Verification items for this drawing (mm, ordinates from the low corner). Coordinates: 2 decimals unless noted, no trailing zeros. Write each loop counter-clockwise with the first axis right and the second up, starting at its lowest first coordinate (ties: lowest second). Pieces come first, ordered by that corner, then holes.
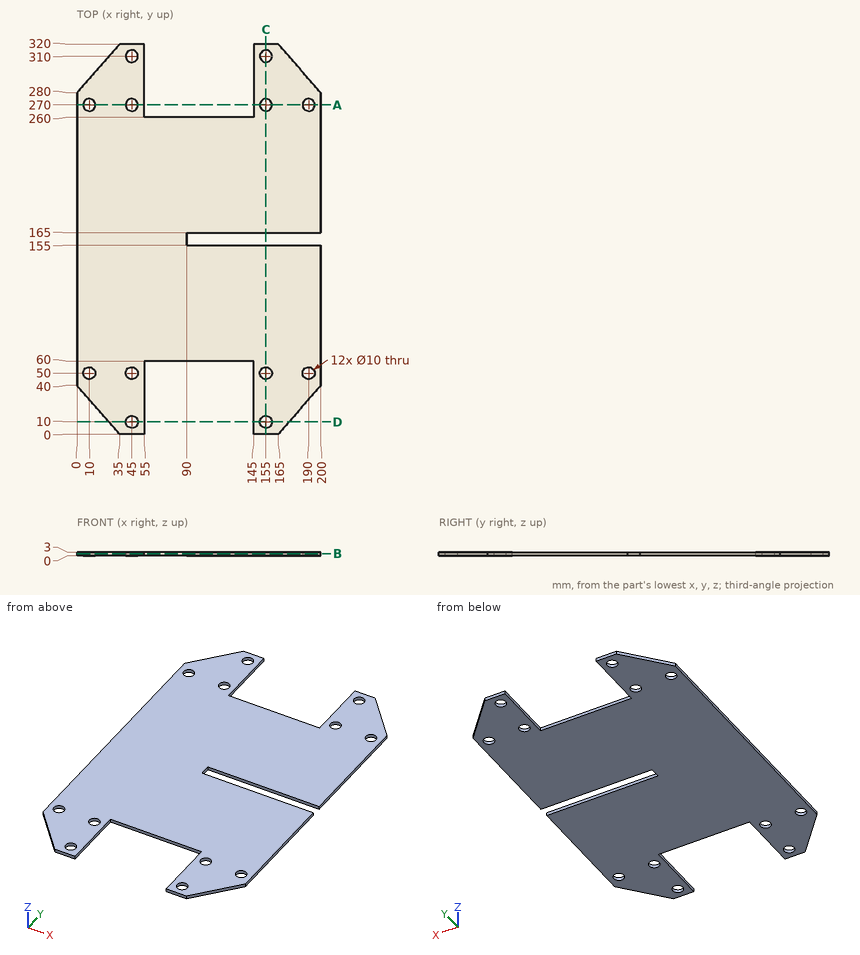
1. Sectioned sample at D-D, the plane y = 10. Record the boundary of the cut face in (x, z).
Computed values:
outline: (26.25, 0) - (40, 0) - (40, 3) - (26.25, 3) - close; (50, 0) - (55, 0) - (55, 3) - (50, 3) - close; (145, 0) - (150, 0) - (150, 3) - (145, 3) - close; (160, 0) - (173.75, 0) - (173.75, 3) - (160, 3) - close
2. Gauge pin test, flat ends, axial feed: pin 1 Ø0.9 at (x, z) = (91, 1) entering from -Y; pin 2 Ø1.5 at (y, z) = (288.5, 1.5) entering from -X. Record the tip position at first contact, or that the pin passes through.
Computed values:
pin 1: stops at y = 60
pin 2: stops at x = 6.78
3. Sectioned sample at B-B, the plane z = 1.8. Give the number of separate pieces and of enclosed holes in the cut face, and give its area (3 significant figures).
Computed values:
separate pieces: 1
enclosed holes: 12
area: 48,400 mm2
4. Sectioned sample at A-A, the plane y = 270. Record the boundary of the cut face in (x, z), and give its area (3 significant figures).
Computed values:
outline: (0, 0) - (5, 0) - (5, 3) - (0, 3) - close; (15, 0) - (40, 0) - (40, 3) - (15, 3) - close; (50, 0) - (55, 0) - (55, 3) - (50, 3) - close; (145, 0) - (150, 0) - (150, 3) - (145, 3) - close; (160, 0) - (185, 0) - (185, 3) - (160, 3) - close; (195, 0) - (200, 0) - (200, 3) - (195, 3) - close
area: 210 mm2
5. Sectioned sample at C-C, the plane x = 155. Record the boundary of the cut face in (y, z).
Computed values:
outline: (0, 0) - (5, 0) - (5, 3) - (0, 3) - close; (15, 0) - (45, 0) - (45, 3) - (15, 3) - close; (55, 0) - (155, 0) - (155, 3) - (55, 3) - close; (165, 0) - (265, 0) - (265, 3) - (165, 3) - close; (275, 0) - (305, 0) - (305, 3) - (275, 3) - close; (315, 0) - (320, 0) - (320, 3) - (315, 3) - close
6. Thickness scan on line 1 along X through (y, z) = (50, 1.35); line 2 along Y through (x, z) = (155, 1.6); line 3 along Y through (x, z) = (190, 1.15). Record the ranges inside material, lowest first.
Computed values:
line 1: x = 0 to 5, 15 to 40, 50 to 55, 145 to 150, 160 to 185, 195 to 200
line 2: y = 0 to 5, 15 to 45, 55 to 155, 165 to 265, 275 to 305, 315 to 320
line 3: y = 28.57 to 45, 55 to 155, 165 to 265, 275 to 291.43
